Design review of the part built by this model. Coordinates are the model's own, in mm. A direction names the side the tool comes from. Round coordinates to 2 decimals unless told otherwise and drop trailing zeros. Write each loop counter-clockwise with the first axis right and the second up, starting at its lowest first coordinate (ties: lowest second). Pieces come first, ordered by that corner, then holes.
from build123d import *

# Parameters (mm, degrees)
SKETCH1_R           = 15
SKETCH1_R_2         = 20
BOSS_EXTRUDE2_DEPTH = 3
BOSS_EXTRUDE4_START = 50
BOSS_EXTRUDE4_DEPTH = 50
SKETCH4_W           = 25
SKETCH4_H           = 12.5
CUT_EXTRUDE1_DEPTH  = 10
FILLET1_R           = 15
SKETCH6_R           = 15
CUT_EXTRUDE2_DEPTH  = 40


with BuildPart() as part:
    # Sketch1 → Boss-Extrude2 (new body)
    with BuildSketch(Plane(origin=(0, 0, 0), x_dir=(1, 0, 0), z_dir=(0, 1, 0))):
        with BuildLine():
            Line((30, 0), (312, 0))
            ThreePointArc((312, 0), (333.213203436, 8.786796564), (342, 30))
            Line((342, 30), (342, 152.5))
            ThreePointArc((342, 152.5), (333.213203436, 173.713203436), (312, 182.5))
            Line((312, 182.5), (30, 182.5))
            ThreePointArc((30, 182.5), (8.786796564, 173.713203436), (0, 152.5))
            Line((0, 152.5), (0, 30))
            ThreePointArc((0, 30), (8.786796564, 8.786796564), (30, 0))
        make_face()
        with Locations(Location((165, 65, 0), (0, 0, 270))):
            Circle(SKETCH1_R, mode=Mode.SUBTRACT)
        with Locations(Location((172, 103.5, 0), (0, 0, 270))):
            Circle(SKETCH1_R, mode=Mode.SUBTRACT)
        with Locations(Location((198, 79, 0), (0, 0, 270))):
            Circle(SKETCH1_R, mode=Mode.SUBTRACT)
        with Locations(Location((205, 117.5, 0), (0, 0, 270))):
            Circle(SKETCH1_R, mode=Mode.SUBTRACT)
        with Locations(Location((234, 79, 0), (0, 0, 270))):
            Circle(SKETCH1_R, mode=Mode.SUBTRACT)
        with Locations(Location((241, 117.5, 0), (0, 0, 270))):
            Circle(SKETCH1_R, mode=Mode.SUBTRACT)
        with Locations(Location((270, 79, 0), (0, 0, 270))):
            Circle(SKETCH1_R, mode=Mode.SUBTRACT)
        with Locations(Location((277, 117.5, 0), (0, 0, 270))):
            Circle(SKETCH1_R, mode=Mode.SUBTRACT)
        with Locations(Location((70, 79, 0), (0, 0, 270))):
            Circle(SKETCH1_R_2, mode=Mode.SUBTRACT)
        with Locations(Location((106, 143.5, 0), (0, 0, 270))):
            Circle(SKETCH1_R, mode=Mode.SUBTRACT)
        with Locations(Location((142, 143.5, 0), (0, 0, 270))):
            Circle(SKETCH1_R, mode=Mode.SUBTRACT)
    extrude(amount=BOSS_EXTRUDE2_DEPTH)

    # Sketch2 → Boss-Extrude4 (add)
    with BuildSketch(Plane.XZ.offset(BOSS_EXTRUDE4_START)):
        with BuildLine():
            Line((30, 0), (312, 0))
            ThreePointArc((312, 0), (333.213203436, -8.786796564), (342, -30))
            Line((342, -30), (342, -152.5))
            ThreePointArc((342, -152.5), (333.213203436, -173.713203436), (312, -182.5))
            Line((312, -182.5), (30, -182.5))
            ThreePointArc((30, -182.5), (8.786796564, -173.713203436), (0, -152.5))
            Line((0, -152.5), (0, -30))
            ThreePointArc((0, -30), (8.786796564, -8.786796564), (30, 0))
        make_face()
        with BuildLine():
            Line((12.5, -30), (12.5, -152.5))
            ThreePointArc((12.5, -152.5), (17.625631329, -164.874368671), (30, -170))
            Line((30, -170), (312, -170))
            ThreePointArc((312, -170), (324.374368671, -164.874368671), (329.5, -152.5))
            Line((329.5, -152.5), (329.5, -30))
            ThreePointArc((329.5, -30), (324.374368671, -17.625631329), (312, -12.5))
            Line((312, -12.5), (30, -12.5))
            ThreePointArc((30, -12.5), (17.625631329, -17.625631329), (12.5, -30))
        make_face(mode=Mode.SUBTRACT)
    extrude(amount=-BOSS_EXTRUDE4_DEPTH)

    # Sketch4 → Cut-Extrude1 (cut)
    with BuildSketch(Plane.XZ.offset(50)):
        with Locations((171, -176.25)):
            Rectangle(SKETCH4_W, SKETCH4_H)
    extrude(amount=-CUT_EXTRUDE1_DEPTH, mode=Mode.SUBTRACT)

    # Fillet1
    fillet1_edges = [part.edges().sort_by_distance(p)[0] for p in [
        (8.786796564, 3, -8.786796564),
        (171, 3, 0),
        (333.213203436, 3, -8.786796564),
        (342, 3, -91.25),
        (333.213203436, 3, -173.713203436),
        (171, 3, -182.5),
        (8.786796564, 3, -173.713203436),
        (0, 3, -91.25),
    ]]
    fillet(fillet1_edges, radius=FILLET1_R)

    # Sketch6 → Cut-Extrude2 (cut)
    with BuildSketch(Plane(origin=(342, 0, 0), x_dir=(0, 0, -1), z_dir=(1, 0, 0))):
        with Locations((127.466870265, -31)):
            Circle(SKETCH6_R)
        with Locations((91.466870265, -31)):
            Circle(SKETCH6_R)
    extrude(amount=-CUT_EXTRUDE2_DEPTH, mode=Mode.SUBTRACT)


solid = part.part
1) For P1, Ø4, axis at x = 165.5, z = -178.5, coming from the -Y side; P2, Ø3, axis at y = -43, z = -178.5, coming from the +X side; P3, Ø18, axis at x = 165, z = -65, coming from the +Y side; P4, Ø5, axis at y = -46.5, z = -179, coming from the -X side, all flat-tipped, find the tip position at first contact; note any pin that passes through.
2) Add section C-C on x = 270. State the section outline as (y, z) points, and give its area (3 significant figures).
3) The part is to be moulded in two halves that separate along Z. For faces 1 (the face through (183.5, -45, -176)), 2 (the face through (9.021, -31.266, -173.945)), 3 (the face through (173, -25, -12.5)), 4 (the face through (17.49, -25.35, -164.74)), say which applies: pulls with the +Z half, pulls with the -Z half, needs draft (parallel to the pull), parting line crosses it, or undercut.
4) For line 1 along Z through (x, y) = (297, -21); line 2 along X through (y, z) = (1.75, -143.5); line 3 along X through (y, z) = (-37.5, -66), list the stretches that pass through material, from the lowest coordinate up.
5) Add section B-B on y = -31. State the section outline as (x, z) points.
6) For faces 5 (the face through (17.76, -25.35, -17.49)), 6 (the face through (335.84, -36.75, -141.32)), 7 (the face through (337.72, -1.51, -92.11)), list the 3-axis set-ups (+Z, -Z, +X, -X, +Y, -Y) from which the entire face can be reached by the end or side of a thin tool; tool diameter is ignored.
7) Add section A-A on x = 106. State the section outline as (y, z) points.
8) Add section D-D on x = 308.5. State the section outline as (y, z) points.
Computed:
1. P1: stops at y = -40
1. P2: stops at x = 329.31
1. P3: passes through
1. P4: stops at x = 12
2. outline: (-50, -182.5) - (-12, -182.5) arc R15 ccw to (3, -167.5) - (3, -130.77) - (0, -130.77) - (0, -170) - (-50, -170) - close; (-50, -12.5) - (0, -12.5) - (0, -64) - (3, -64) - (3, -15) arc R15 ccw to (-12, 0) - (-50, 0) - close; (0, -104.23) - (3, -104.23) - (3, -94) - (0, -94) - close
2. area: 1,530 mm2
3. face 1: needs draft
3. face 2: pulls with the -Z half
3. face 3: undercut
3. face 4: undercut
4. line 1: z = -182.5 to -170, -12.5 to 0
4. line 2: x = 9.01 to 91, 121 to 127, 157 to 332.99
4. line 3: x = 0 to 12.5, 329.5 to 342
5. outline: (0, -152.5) arc R30 ccw to (30, -182.5) - (312, -182.5) arc R30 ccw to (342, -152.5) - (342, -142.47) - (329.5, -142.47) - (329.5, -152.5) arc R17.5 cw to (312, -170) - (30, -170) arc R17.5 cw to (12.5, -152.5) - (12.5, -30) arc R17.5 cw to (30, -12.5) - (312, -12.5) arc R17.5 cw to (329.5, -30) - (329.5, -76.47) - (342, -76.47) - (342, -30) arc R30 ccw to (312, 0) - (30, 0) arc R30 ccw to (0, -30) - close; (329.5, -112.47) - (342, -112.47) - (342, -106.47) - (329.5, -106.47) - close
6. face 5: -Y
6. face 6: +X
6. face 7: +Z, -Z, +X, +Y
7. outline: (-50, -182.5) - (-12, -182.5) arc R15 ccw to (3, -167.5) - (3, -158.5) - (0, -158.5) - (0, -170) - (-50, -170) - close; (-50, -12.5) - (0, -12.5) - (0, -128.5) - (3, -128.5) - (3, -15) arc R15 ccw to (-12, 0) - (-50, 0) - close
8. outline: (-50, -182.5) - (-12, -182.5) arc R15 ccw to (3, -167.5) - (3, -15) arc R15 ccw to (-12, 0) - (-50, 0) - (-50, -12.5) - (0, -12.5) - (0, -170) - (-50, -170) - close
